Could you check a few things on this model? Use its own coordinates, in mm. A direction names the side the tool comes from. Coordinates: 2 decimals unless noted, no trailing zeros. Loops run counter-clockwise (first coordinate to the right, second up) from the corner with the lowest first, then second, coordinate; pieces in that order, holes last. Notation, with made-up numbers: (74, -13) - (84, -13) arc R24 cw to (84, -3) - close; hole circle Ø2 at (-32.5, 24). An arc over 180 degrees is marked (long way). One line per question, with ' | ' between items. Start each with the question number.
1. I want a section at C-C, the plane x = -105. Write out the boundary of the cut face in (y, z).
2. I want a section at B-B, the plane z = -79. Write out the boundary of the cut face in (x, y).
3. I want a section at A-A, the plane x = 8. Write out the boundary of the cut face in (y, z), then the cut area to 3 significant figures.
4. We'd pull the mould along X, two halves only. Please class faces 1 (the cylindrical face through (-35.91, 1.97, -8.08)), 2 (the flat face through (-20, 4, -43)): pulls with the +X half, pulls with the -X half, needs draft (parallel to the pull), parting line crosses it, or undercut.
5. Which directions (+Z, -Z, +X, -X, +Y, -Y) give clear straight access to the entire face, cutting with the end or side of a thin tool? Please do faces 3 (the flat face through (-20, 0, -43)), 4 (the cylindrical face through (-35.91, 1.97, -43.08)).
6. Please list where these lines run through material, in increasing order: L1, parallel to Z at x = -118, y = 1.05; L2, parallel to Z at x = 23.5, y = 2.1; L3, parallel to X at y = 0.5, z = -78.5. Write a range as [from, to].
7. I'm going to push flat-ended pins straight in: P1, Ø1, axis at x = -46, y = 1.5, coming from the +Z side; P2, Ø2, axis at x = 76, y = 2.5, coming from the -Z side. Where does each tip first touch, or does it pass through?
8. I want a section at D-D, the plane y = 0.95. Count the separate pieces of the cut face and the enclosed holes in it, then the cut area to 3 significant figures.
from build123d import *

# Parameters (mm, degrees)
BOSS_EXTRUDE1_DEPTH = 4


with BuildPart() as part:
    # Sketch1 → Boss-Extrude1 (new body)
    with BuildSketch(Plane(origin=(0, 0, 0), x_dir=(1, 0, 0), z_dir=(0, 1, 0))):
        Polygon((-69.534910804, 105.258653628), (-49.534910804, 105.258653628), (-49.534910804, 100.258653628), (5.503649635, 100.258653628), (5.465089196, 105.258653628), (25.465089196, 105.258653628), (25.465089196, 100.258653628), (80.465089196, 100.258653628), (80.465089196, 105.258653628), (100.465089196, 105.258653628), (100.465089196, 100.258653628), (100.465089196, -15.741346372), (100.465089196, -20.741346372), (80.465089196, -20.741346372), (80.465089196, -15.741346372), (25.465089196, -15.741346372), (25.465089196, -20.741346372), (5.465089196, -20.741346372), (5.503649635, -15.741346372), (-49.534910804, -15.741346372), (-49.534910804, -20.741346372), (-69.534910804, -20.741346372), (-69.496350365, -15.741346372), (-124.534910804, -15.741346372), (-124.534910804, -20.741346372), (-144.534910804, -20.741346372), (-144.534910804, 105.258653628), (-124.534910804, 105.258653628), (-124.534910804, 100.258653628), (-69.496350365, 100.258653628), align=None)
        with BuildLine():
            Line((-4.534910804, 86.514295241), (75.465089196, 86.514295241))
            ThreePointArc((75.465089196, 86.514295241), (84.091672485, 77.887711952), (75.465089196, 69.261128664))
            Line((75.465089196, 69.261128664), (-4.534910804, 69.261128664))
            ThreePointArc((-4.534910804, 69.261128664), (-13.161494092, 77.887711952), (-4.534910804, 86.514295241))
        make_face(mode=Mode.SUBTRACT)
        with BuildLine():
            Line((-124.534910804, 86.514295241), (-44.534910804, 86.514295241))
            ThreePointArc((-44.534910804, 86.514295241), (-35.908327515, 77.887711952), (-44.534910804, 69.261128664))
            Line((-44.534910804, 69.261128664), (-124.534910804, 69.261128664))
            ThreePointArc((-124.534910804, 69.261128664), (-133.161494092, 77.887711952), (-124.534910804, 86.514295241))
        make_face(mode=Mode.SUBTRACT)
        with BuildLine():
            Line((-4.534910804, 51.514295241), (75.465089196, 51.514295241))
            ThreePointArc((75.465089196, 51.514295241), (84.091672485, 42.887711952), (75.465089196, 34.261128664))
            Line((75.465089196, 34.261128664), (-4.534910804, 34.261128664))
            ThreePointArc((-4.534910804, 34.261128664), (-13.161494092, 42.887711952), (-4.534910804, 51.514295241))
        make_face(mode=Mode.SUBTRACT)
        with BuildLine():
            Line((-4.534910804, 16.514295241), (75.465089196, 16.514295241))
            ThreePointArc((75.465089196, 16.514295241), (84.091672485, 7.887711952), (75.465089196, -0.738871336))
            Line((75.465089196, -0.738871336), (-4.534910804, -0.738871336))
            ThreePointArc((-4.534910804, -0.738871336), (-13.161494092, 7.887711952), (-4.534910804, 16.514295241))
        make_face(mode=Mode.SUBTRACT)
        with BuildLine():
            Line((-124.534910804, 51.514295241), (-44.534910804, 51.514295241))
            ThreePointArc((-44.534910804, 51.514295241), (-35.908327515, 42.887711952), (-44.534910804, 34.261128664))
            Line((-44.534910804, 34.261128664), (-124.534910804, 34.261128664))
            ThreePointArc((-124.534910804, 34.261128664), (-133.161494092, 42.887711952), (-124.534910804, 51.514295241))
        make_face(mode=Mode.SUBTRACT)
        with BuildLine():
            Line((-124.534910804, 16.514295241), (-44.534910804, 16.514295241))
            ThreePointArc((-44.534910804, 16.514295241), (-35.908327515, 7.887711952), (-44.534910804, -0.738871336))
            Line((-44.534910804, -0.738871336), (-124.534910804, -0.738871336))
            ThreePointArc((-124.534910804, -0.738871336), (-133.161494092, 7.887711952), (-124.534910804, 16.514295241))
        make_face(mode=Mode.SUBTRACT)
    extrude(amount=BOSS_EXTRUDE1_DEPTH)


solid = part.part
Results are:
1) outline: (0, -100.26) - (4, -100.26) - (4, -86.51) - (0, -86.51) - close; (0, -69.26) - (4, -69.26) - (4, -51.51) - (0, -51.51) - close; (0, -34.26) - (4, -34.26) - (4, -16.51) - (0, -16.51) - close; (0, 0.74) - (4, 0.74) - (4, 15.74) - (0, 15.74) - close
2) outline: (-144.53, 0) - (-133.09, 0) - (-133.09, 4) - (-144.53, 4) - close; (-35.98, 0) - (-13.09, 0) - (-13.09, 4) - (-35.98, 4) - close; (84.02, 0) - (100.47, 0) - (100.47, 4) - (84.02, 4) - close
3) outline: (0, -105.26) - (4, -105.26) - (4, -86.51) - (0, -86.51) - close; (0, -69.26) - (4, -69.26) - (4, -51.51) - (0, -51.51) - close; (0, -34.26) - (4, -34.26) - (4, -16.51) - (0, -16.51) - close; (0, 0.74) - (4, 0.74) - (4, 20.74) - (0, 20.74) - close | area: 297 mm2
4) face 1: undercut | face 2: needs draft
5) face 3: +Z, -Z, +X, -X, -Y | face 4: +Y, -Y
6) L1: z = [-100.26, -86.51], [-69.26, -51.51], [-34.26, -16.51], [0.74, 15.74] | L2: z = [-105.26, -86.51], [-69.26, -51.51], [-34.26, -16.51], [0.74, 20.74] | L3: x = [-144.53, -133.14], [-35.93, -13.14], [84.07, 100.47]
7) P1: stops at z = 15.74 | P2: stops at z = -100.26
8) separate pieces: 1 | enclosed holes: 6 | area: 19,500 mm2
